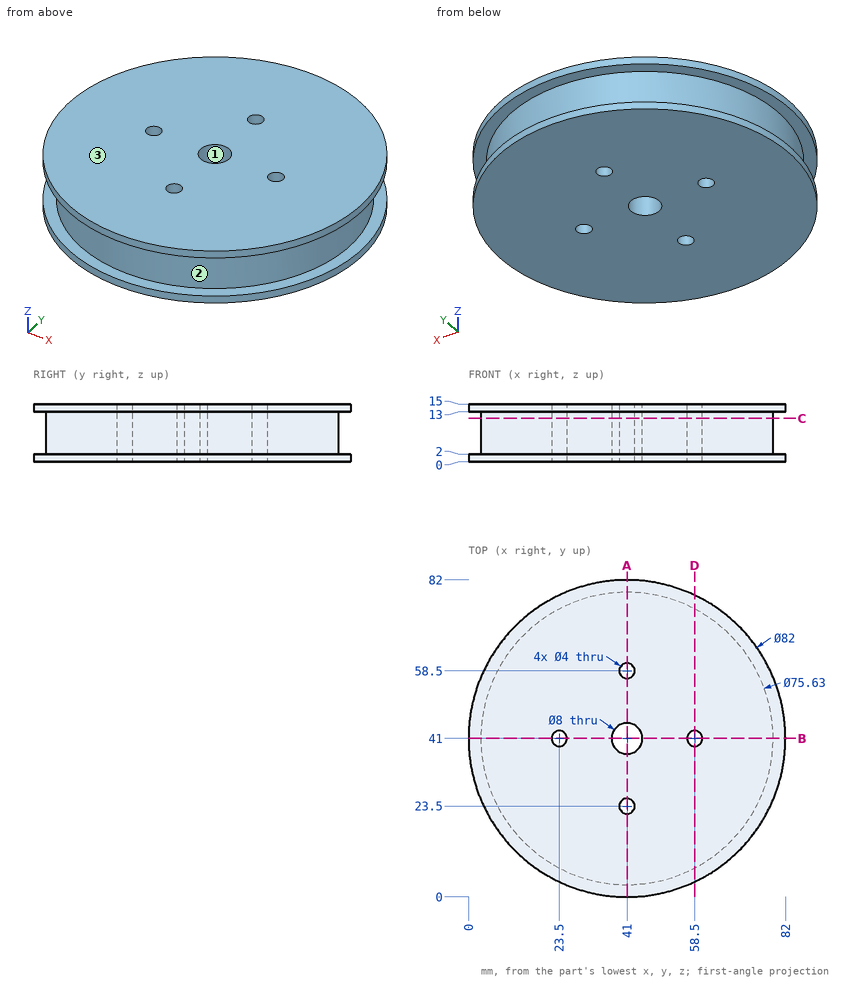
Drawing for the job (mm, zero at the part's lowest x, y, z). Give positions to 0.01 mm unless a question says otherwise; leave off trailing zeros. Order: outer loops, then holes, each group sorted by start corner. A loop starts at its lowest first (then second) coordinate and runs counter-clockwise, first axis right, second up. Notation, with made-up numbers: M 6,63 L 46,63 A14 cw 46,81 Z; hole C -17,10.25 d7. An arc over 180 degrees is marked long. Use a Markdown table: item, result. Add a question column.
(1) Mould opens along X. For the marked faces 1, 2 and 3 say: +X half, -X half, draft (parallel to the pull), parting line (faces both ways), or undercut.
(2) Saw through at C-C, the plane z = 11.25. Give the cut face in (x, y) (3 decimals), and give its area (3 significant figures).
(3) Probe line 1 along Y through (x, z) = (41, 4.75) (3 decimals); line 2 along Z through (x, y) = (62.5, 73.5); line 3 along X through (y, z) = (59, 4). List the from-to ranges inside material, lowest first. Write a range as [from, to].
(4) Saw through at D-D, the plane x = 58.5. Give the cut face in (y, z).
(5) Drop flat-ended pins along their axis: P1, Ø1, axis at x = 25, z = 11, coming from the +Y side; P2, Ø8, axis at y = 57, z = 12, coming from the +X side; P3, Ø1, axis at x = 71, z = 9.5, coming from the +Y side. Give the stop position or say it passes through.
(6) Saw through at A-A, the plane x = 41. Give the cut face in (y, z) (3 decimals).
Answer key:
| question | item | result |
|---|---|---|
| 1 | face 1 | undercut |
| 1 | face 2 | parting line |
| 1 | face 3 | draft |
| 2 | outline | C 41,41 d75.63; hole C 23.5,41 d4; hole C 41,41 d8; hole C 41,23.5 d4; hole C 41,58.5 d4; hole C 58.5,41 d4 |
| 2 | area | 4,390 mm^2 |
| 3 | line 1 | [3.185, 21.5], [25.5, 37], [45, 56.5], [60.5, 78.815] |
| 3 | line 2 | [0, 2], [13, 15] |
| 3 | line 3 | [7.74, 39.06], [42.94, 74.26] |
| 4 | outline | M 3.92,0 L 39,0 L 39,15 L 3.92,15 L 3.92,13 L 7.48,13 L 7.48,2 L 3.92,2 Z; M 43,0 L 78.08,0 L 78.08,2 L 74.52,2 L 74.52,13 L 78.08,13 L 78.08,15 L 43,15 Z |
| 5 | P1 | y = 75.49 |
| 5 | P2 | x = 80.17 |
| 5 | P3 | y = 64.66 |
| 6 | outline | M 0,0 L 21.5,0 L 21.5,15 L 0,15 L 0,13 L 3.185,13 L 3.185,2 L 0,2 Z; M 25.5,0 L 37,0 L 37,15 L 25.5,15 Z; M 45,0 L 56.5,0 L 56.5,15 L 45,15 Z; M 60.5,0 L 82,0 L 82,2 L 78.815,2 L 78.815,13 L 82,13 L 82,15 L 60.5,15 Z |
